```python
from build123d import *

# Parameters (mm, degrees)
F0_W     = 58
F0_H     = 28
F0_W_2   = 55
F0_H_2   = 25
F0_W_3   = 53
F0_H_3   = 23
F0_W_4   = 50
F0_H_4   = 20
F1_DEPTH = 1.5
F2_DEPTH = 1.5
F3_SIZE  = 1.49999


# Not quite as in the source:
# - a fillet or chamfer is up to 0.001 mm smaller than in the source, because OpenCascade refuses the exact size


with BuildPart() as f1:
    # F0 (on Top) → F1 (new body)
    with BuildSketch(Plane.XY):
        Rectangle(F0_W, F0_H)
        Rectangle(F0_W_2, F0_H_2, mode=Mode.SUBTRACT)
        Rectangle(F0_W_2, F0_H_2)
        Rectangle(F0_W_3, F0_H_3, mode=Mode.SUBTRACT)
        Rectangle(F0_W_3, F0_H_3)
        Rectangle(F0_W_4, F0_H_4, mode=Mode.SUBTRACT)
    extrude(amount=-F1_DEPTH)

    # F0 (on Top) → F2 (join)
    with BuildSketch(Plane.XY):
        Rectangle(F0_W_2, F0_H_2)
        Rectangle(F0_W_3, F0_H_3, mode=Mode.SUBTRACT)
    extrude(amount=F2_DEPTH)

    # F3 (size 1.5 in the source; OpenCascade refuses exactly that, so slightly less here)
    f3_edges = [f1.edges().sort_by_distance(p)[0] for p in [
        (0, -14, -1.5),
        (-29, 0, -1.5),
        (0, 14, -1.5),
        (29, 0, -1.5),
    ]]
    chamfer(f3_edges, length=F3_SIZE)


solid = f1.part
```
Source: CAD feature listing. Evaluate the final solid. Frame: model axes, mm. A direction names the side the tool comes from. Coordinates: 2 decimals unless noted, no trailing zeros. Write each loop counter-clockwise with the first axis right and the second up, starting at its lowest first coordinate (ties: lowest second). Pieces come first, ordered by that corner, then holes. Notation, with made-up numbers: (-15.75, -31) -> (35.25, -31) arc R26 cw to (35.25, 7) -> close; hole circle Ø8 at (47, 49). An arc over 180 degrees is marked (long way). Return JSON: item names as keys, results as strings. Group by question number.
1) Mould query, pull axis Y, two halves, no side actions, for faces 5 (the face through (0, 10, -1)), 6 (the face through (-28, 0, -1)), 7 (the face through (0, -12.5, 1)). Classes: +Y half, -Y half, draft (parallel to the pull), parting line (faces both ways), or undercut.
2) Ray query, line 1 along X through (y, z) = (2.5, 1.3); line 2 along Y through (x, z) = (3, 1.2); line 3 along Z through (x, y) = (16, -10.25). Return the intervals inside material, ascending.
3) Section query C-C, the plane z = 1. Return loops of the section in (x, y), plus the area to 3 significant figures.
4) Contact query for flat-ended pins moving along their axis: P1, Ø0.8, axis at y = -5, z = 1, coming from the +X side; P2, Ø8, axis at x = 13.5, y = -6.5, coming from the +Z side; P3, Ø1.6, axis at x = 0.5, z = 1, coming from the +Y side. Output: stop coordinate, or through.
5) Set-up query: faces 1 (the face through (0, -11.5, 1)), 2 (the face through (27.5, 0, 1)), 3 (the face through (-27.5, 0, 1)), 4 (the face through (-25, 0, -1)). Return all of +Z, -Z, +X, -X, +Y, -Y with unobstructed straight access to the full face (end or side cutting, diameter ignored); none if empty.
From the geometry:
{
 "1": {"face 5": "undercut", "face 6": "draft", "face 7": "-Y half"},
 "2": {"line 1": "-27.5 to -26.5, 26.5 to 27.5", "line 2": "-12.5 to -11.5, 11.5 to 12.5", "line 3": "-1.5 to 0"},
 "3": {"outline": "(-27.5, -12.5) -> (27.5, -12.5) -> (27.5, 12.5) -> (-27.5, 12.5) -> close; hole (-26.5, -11.5) -> (26.5, -11.5) -> (26.5, 11.5) -> (-26.5, 11.5) -> close", "area": "156 mm²"},
 "4": {"P1": "x = 27.5", "P2": "z = 0", "P3": "y = 12.5"},
 "5": {"face 1": "+Z", "face 2": "+Z, +X, +Y, -Y", "face 3": "+Z, -X, +Y, -Y", "face 4": "+Z, -Z"}
}
